```python
from build123d import *

# Parameters (mm, degrees)
SKETCH1_W           = 42
SKETCH1_H           = 42
BOSS_EXTRUDE1_DEPTH = 26
CHAMFER1_SIZE       = 3
SKETCH4_R           = 11.25
BOSS_EXTRUDE2_DEPTH = 0.5
CUT_EXTRUDE4_REACH  = 41.472
SKETCH8_R           = 1.5
SKETCH9_R           = 18.35
CUT_EXTRUDE5_DEPTH  = 0.5
SKETCH10_R          = 8.9
SKETCH10_R_2        = 2.75
BOSS_EXTRUDE3_DEPTH = 3.5
BOSS_EXTRUDE4_DEPTH = 26.3
FILLET1_R           = 0.5


with BuildPart() as part:
    # Sketch1 → Boss-Extrude1 (new body)
    with BuildSketch(Plane.XY):
        Rectangle(SKETCH1_W, SKETCH1_H)
    extrude(amount=BOSS_EXTRUDE1_DEPTH)

    # Chamfer1
    chamfer1_edges = [part.edges().sort_by_distance(p)[0] for p in [
        (-21, 21, 13),
        (21, 21, 13),
        (21, -21, 13),
        (-21, -21, 13),
    ]]
    chamfer(chamfer1_edges, length=CHAMFER1_SIZE)

    # Sketch4 → Boss-Extrude2 (add)
    with BuildSketch(Plane(origin=(0, 0, 0), x_dir=(-1, 0, 0), z_dir=(0, 0, -1))):
        Circle(SKETCH4_R)
    extrude(amount=-BOSS_EXTRUDE2_DEPTH)

    # Sketch8 → Cut-Extrude4 (cut, up to next)
    with BuildSketch(Plane(origin=(0, 0, 0), x_dir=(-1, 0, 0), z_dir=(0, 0, -1)), mode=Mode.PRIVATE) as cut_extrude4_sk1:
        with Locations((15.5, 15.5)):
            Circle(SKETCH8_R)
    cut_extrude4_tool1 = extrude(cut_extrude4_sk1.sketch, amount=-CUT_EXTRUDE4_REACH, mode=Mode.PRIVATE) & part.part
    # Sketch8 → Cut-Extrude4 (cut, up to next)
    with BuildSketch(Plane(origin=(0, 0, 0), x_dir=(-1, 0, 0), z_dir=(0, 0, -1)), mode=Mode.PRIVATE) as cut_extrude4_sk2:
        with Locations((-15.5, 15.5)):
            Circle(SKETCH8_R)
    cut_extrude4_tool2 = extrude(cut_extrude4_sk2.sketch, amount=-CUT_EXTRUDE4_REACH, mode=Mode.PRIVATE) & part.part
    # Sketch8 → Cut-Extrude4 (cut, up to next)
    with BuildSketch(Plane(origin=(0, 0, 0), x_dir=(-1, 0, 0), z_dir=(0, 0, -1)), mode=Mode.PRIVATE) as cut_extrude4_sk3:
        with Locations((-15.5, -15.5)):
            Circle(SKETCH8_R)
    cut_extrude4_tool3 = extrude(cut_extrude4_sk3.sketch, amount=-CUT_EXTRUDE4_REACH, mode=Mode.PRIVATE) & part.part
    # Sketch8 → Cut-Extrude4 (cut, up to next)
    with BuildSketch(Plane(origin=(0, 0, 0), x_dir=(-1, 0, 0), z_dir=(0, 0, -1)), mode=Mode.PRIVATE) as cut_extrude4_sk4:
        with Locations((15.5, -15.5)):
            Circle(SKETCH8_R)
    cut_extrude4_tool4 = extrude(cut_extrude4_sk4.sketch, amount=-CUT_EXTRUDE4_REACH, mode=Mode.PRIVATE) & part.part
    add(cut_extrude4_tool1.solids().sort_by_distance((-15.5, 15.5, 0))[0], mode=Mode.SUBTRACT)
    add(cut_extrude4_tool2.solids().sort_by_distance((15.5, 15.5, 0))[0], mode=Mode.SUBTRACT)
    add(cut_extrude4_tool3.solids().sort_by_distance((15.5, -15.5, 0))[0], mode=Mode.SUBTRACT)
    add(cut_extrude4_tool4.solids().sort_by_distance((-15.5, -15.5, 0))[0], mode=Mode.SUBTRACT)

    # Sketch9 → Cut-Extrude5 (cut)
    with BuildSketch(Plane(origin=(0, 0, 0), x_dir=(-1, 0, 0), z_dir=(0, 0, -1))):
        Circle(SKETCH9_R)
    extrude(amount=-CUT_EXTRUDE5_DEPTH, mode=Mode.SUBTRACT)

    # Sketch10 → Boss-Extrude3 (add)
    with BuildSketch(Plane(origin=(0, 0, 0.5), x_dir=(-1, 0, 0), z_dir=(0, 0, -1))):
        with Locations((0, 8.3)):
            Circle(SKETCH10_R)
        with Locations((0, 8.3)):
            Circle(SKETCH10_R_2, mode=Mode.SUBTRACT)
    extrude(amount=BOSS_EXTRUDE3_DEPTH)

    # Sketch11 → Boss-Extrude4 (add)
    with BuildSketch(Plane(origin=(0, 0, 0.5), x_dir=(-1, 0, 0), z_dir=(0, 0, -1))):
        with BuildLine():
            Line((-1.681517172, 6.45), (1.681517172, 6.45))
            ThreePointArc((1.681517172, 6.45), (0, 10.8), (-1.681517172, 6.45))
        make_face()
    extrude(amount=BOSS_EXTRUDE4_DEPTH)

    # Fillet1
    fillet1_edges = [part.edges().sort_by_distance(p)[0] for p in [
        (8.9, 8.3, 0.5),
    ]]
    fillet(fillet1_edges, radius=FILLET1_R)


solid = part.part
```
CAD build for the part. Positions are in the model's coordinates, mm. A direction names the side the tool comes from. Round coordinates to 2 decimals unless told otherwise and drop trailing zeros. Loops run counter-clockwise (first coordinate to the right, second up) from the corner with the lowest first, then second, coordinate; pieces in that order, holes last. Notation, with made-up numbers: M 76,50.5 L 91,50.5 A7 ccw 91,56.5 Z; hole C 74,53.5 d2. An arc over 180 degrees is marked long. Return JSON: item names as keys, results as strings. Group by question number.
(1) Tool access for faces 1 (the flat face through (21, 0, 13)), 2 (the cylindrical face through (1.159, 17.124, -1.479)): list every direction of +Z, -Z, +X, -X, +Y, -Y with a clear straight run to the whole face (end or side of a thin tool).
(2) Saw through at B-B, the plane z = -2. List the corners of the cut face in (x, y), and give its area (3 significant figures).
(3) Wall check: probe 1 along Y at (x, z) = (-15.5, 18.75); probe 2 along X at (y, z) = (-15, 8); probe 3 along Z at (x, y) = (4, -13.5). Give the ranges that are in metal, low to high. Write a range as [from, to].
(4) Saw through at C-C, the plane x = -15.5. List the corners of the cut face in (y, z), and give its area (3 significant figures).
(5) Drop flat-ended pins along their axis: P1, Ø1, axis at x = 2, y = -13.5, coming from the -Z side; P2, Ø2, axis at x = -2, y = -0.5, coming from the -Z side; P3, Ø5.5, axis at x = -2.5, y = 11.5, coming from the -Z side; P4, Ø3.5, axis at x = 15.5, y = 15.5, coming from the -Z side. Give the stop position or say it passes through.
(6) Mould opens along X. For faces 3 (the flat face through (20, -19, 13)), 4 (the flat face through (-21, 0, 13)), 5 (the cylindrical face through (17, -15.43, 12.82)) say: +X half, -X half, draft (parallel to the pull), parting line (faces both ways), or undercut.
(7) Saw through at A-A, the plane z = 8. List the corners of the cut face in (x, y), and give its area (3 significant figures).
Answer list:
{
 "1": {"face 1": "+Z, -Z, +X, +Y, -Y", "face 2": "-Z"},
 "2": {"outline": "C 0,8.3 d17.8; M -1.68,6.45 L 1.68,6.45 A2.5 ccw long Z; hole C 0,8.3 d5.5", "area": "243 mm2"},
 "3": {"probe 1": "[-21, -17], [-14, 14], [17, 21]", "probe 2": "[-21, -16.91], [-14.09, 14.09], [16.91, 21]", "probe 3": "[0.5, 26]"},
 "4": {"outline": "M -21,0 L -17,0 L -17,26 L -21,26 Z; M -14,0 L -9.82,0 L -9.82,0.5 L 9.82,0.5 L 9.82,0 L 14,0 L 14,26 L -14,26 Z; M 17,0 L 21,0 L 21,26 L 17,26 Z", "area": "926 mm2"},
 "5": {"P1": "z = 0.5", "P2": "z = -3", "P3": "z = -25.8", "P4": "z = 0"},
 "6": {"face 3": "+X half", "face 4": "-X half", "face 5": "undercut"},
 "7": {"outline": "M -21,-18 L -18,-21 L 18,-21 L 21,-18 L 21,18 L 18,21 L -18,21 L -21,18 Z; hole C -15.5,-15.5 d3; hole C -15.5,15.5 d3; hole C 15.5,-15.5 d3; hole C 15.5,15.5 d3", "area": "1,720 mm2"}
}
